Part model, mm, in its own coordinate system. Give positions to 0.01 mm unless a question says otherwise; leave off trailing zeros. Order: outer loops, then holes, each group sorted by start corner. A loop starts at its lowest first (then second) coordinate and runs counter-clockwise, first axis right, second up. Notation, with made-up numbers: M 45.25,28.5 L 52.25,28.5 A32 cw 52.25,64.5 Z; hole C 72,3 d10. An arc over 180 degrees is marked long. One line per question, with ' | ' between items.
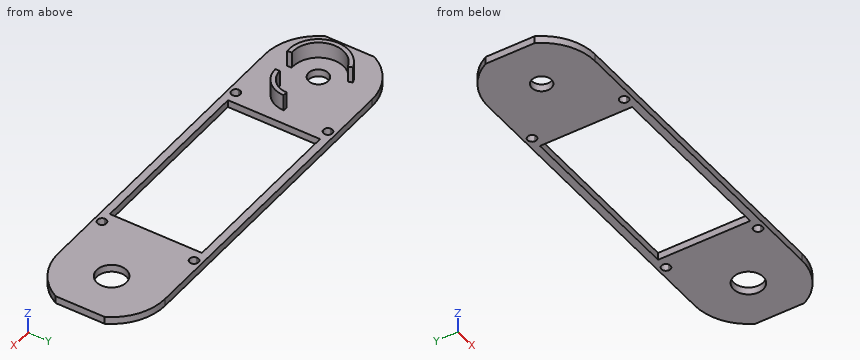
```python
from build123d import *

# Parameters (mm, degrees)
F0_R     = 30
F0_R_2   = 10
F0_R_3   = 14
F0_R_4   = 6.6
F1_DEPTH = 5
F3_DEPTH = 11


with BuildPart() as f1:
    # F0 (on Top) → F1 (new body)
    with BuildSketch(Plane.XY):
        with BuildLine():
            ThreePointArc((18.3030052177, -31), (31.2642622481, -17.8478543831), (36, 0))
            ThreePointArc((36, 0), (31.2978497092, 17.7888898917), (18.4197442455, 30.9307779069))
            ThreePointArc((18.4197442455, 30.9307779069), (9.5522770937, 34.7095664382), (0, 36))
            ThreePointArc((0, 36), (-18.7386337537, 30.7386337537), (-32, 16.4924225025))
            Line((-32, 16.4924225025), (-32, -16.4924225025))
            ThreePointArc((-32, -16.4924225025), (-18.7386337537, -30.7386337537), (0, -36))
            ThreePointArc((0, -36), (9.4868329805, -34.7275107084), (18.3030052177, -31))
        make_face()
        Circle(F0_R, mode=Mode.SUBTRACT)
        with BuildLine():
            ThreePointArc((242, 16.4924225025), (228.7386337537, 30.7386337537), (210, 36))
            ThreePointArc((210, 36), (200.4477229063, 34.7095664382), (191.5802557545, 30.9307779069))
            ThreePointArc((191.5802557545, 30.9307779069), (174.0000639573, -0.0678595955), (191.6969947823, -31))
            ThreePointArc((191.6969947823, -31), (200.5131670195, -34.7275107084), (210, -36))
            ThreePointArc((210, -36), (228.7386337537, -30.7386337537), (242, -16.4924225025))
            Line((242, -16.4924225025), (242, 16.4924225025))
        make_face()
        with Locations((210, 0)):
            Circle(F0_R, mode=Mode.SUBTRACT)
        Circle(F0_R)
        Circle(F0_R_2, mode=Mode.SUBTRACT)
        with Locations((210, 0)):
            Circle(F0_R)
        with Locations((210, 0)):
            Circle(F0_R_3, mode=Mode.SUBTRACT)
        with BuildLine():
            ThreePointArc((19.6214168703, 36), (23.4046464655, 33.6633706545), (26.9125802938, 30.9307779069))
            Line((26.9125802938, 30.9307779069), (34, 30.9307779069))
            ThreePointArc((34, 30.9307779069), (37, 33.9307779069), (40, 30.9307779069))
            Line((40, 30.9307779069), (45, 30.9307779069))
            Line((45, 30.9307779069), (165, 30.9307779069))
            Line((165, 30.9307779069), (170, 30.9307779069))
            ThreePointArc((170, 30.9307779069), (173, 33.9307779069), (176, 30.9307779069))
            Line((176, 30.9307779069), (183.0874197062, 30.9307779069))
            ThreePointArc((183.0874197062, 30.9307779069), (186.5953535345, 33.6633706545), (190.3785831296, 36))
            Line((190.3785831296, 36), (19.6214168703, 36))
        make_face()
        with BuildLine():
            Line((34, -31), (26.83281573, -31))
            ThreePointArc((26.83281573, -31), (23.361269906, -33.693487032), (19.6214168703, -36))
            Line((19.6214168703, -36), (190.3785831296, -36))
            ThreePointArc((190.3785831296, -36), (186.638730094, -33.693487032), (183.16718427, -31))
            Line((183.16718427, -31), (176, -31))
            ThreePointArc((176, -31), (173, -34), (170, -31))
            Line((170, -31), (165, -31))
            Line((165, -31), (45, -31))
            Line((45, -31), (40, -31))
            ThreePointArc((40, -31), (37, -34), (34, -31))
        make_face()
        with Locations((210, 0)):
            Circle(F0_R_3)
        with Locations((210, 0)):
            Circle(F0_R_2, mode=Mode.SUBTRACT)
        with BuildLine():
            Line((37, 27.9307779069), (37, 17.6635217327))
            ThreePointArc((37, 17.6635217327), (39.9874980463, 9.0553851381), (41, 0))
            ThreePointArc((41, 0), (39.9874980463, -9.0553851381), (37, -17.6635217327))
            Line((37, -17.6635217327), (37, -28))
            ThreePointArc((37, -28), (39.1213203436, -28.8786796564), (40, -31))
            Line((40, -31), (45, -31))
            Line((45, -31), (45, 30.9307779069))
            Line((45, 30.9307779069), (40, 30.9307779069))
            ThreePointArc((40, 30.9307779069), (39.1213203436, 28.8094575634), (37, 27.9307779069))
        make_face()
        with BuildLine():
            ThreePointArc((173, -17.6635217327), (169, 0), (173, 17.6635217327))
            Line((173, 17.6635217327), (173, 27.9307779069))
            ThreePointArc((173, 27.9307779069), (170.8786796564, 28.8094575634), (170, 30.9307779069))
            Line((170, 30.9307779069), (165, 30.9307779069))
            Line((165, 30.9307779069), (165, -31))
            Line((165, -31), (170, -31))
            ThreePointArc((170, -31), (170.8786796564, -28.8786796564), (173, -28))
            Line((173, -28), (173, -17.6635217327))
        make_face()
        Circle(F0_R_2)
        Circle(F0_R_4, mode=Mode.SUBTRACT)
        with BuildLine():
            ThreePointArc((18.4197442455, 30.9307779069), (31.2978497092, 17.7888898917), (36, 0))
            ThreePointArc((36, 0), (31.2642622481, -17.8478543831), (18.3030052177, -31))
            Line((18.3030052177, -31), (26.83281573, -31))
            ThreePointArc((26.83281573, -31), (32.6055594055, -24.8571417474), (37, -17.6635217327))
            Line((37, -17.6635217327), (37, 17.6635217327))
            ThreePointArc((37, 17.6635217327), (32.6375474194, 24.815126404), (26.9125802938, 30.9307779069))
            Line((26.9125802938, 30.9307779069), (18.4197442455, 30.9307779069))
        make_face()
        with BuildLine():
            Line((191.5802557545, 30.9307779069), (183.0874197062, 30.9307779069))
            ThreePointArc((183.0874197062, 30.9307779069), (177.3624525806, 24.815126404), (173, 17.6635217327))
            Line((173, 17.6635217327), (173, -17.6635217327))
            ThreePointArc((173, -17.6635217327), (177.3944405945, -24.8571417474), (183.16718427, -31))
            Line((183.16718427, -31), (191.6969947823, -31))
            ThreePointArc((191.6969947823, -31), (174.0000639573, -0.0678595955), (191.5802557545, 30.9307779069))
        make_face()
        with BuildLine():
            ThreePointArc((41, 0), (39.9874980463, 9.0553851381), (37, 17.6635217327))
            Line((37, 17.6635217327), (37, -17.6635217327))
            ThreePointArc((37, -17.6635217327), (39.9874980463, -9.0553851381), (41, 0))
        make_face()
        with BuildLine():
            Line((173, -17.6635217327), (173, 17.6635217327))
            ThreePointArc((173, 17.6635217327), (169, 0), (173, -17.6635217327))
        make_face()
        with BuildLine():
            ThreePointArc((0, 36), (9.5522770937, 34.7095664382), (18.4197442455, 30.9307779069))
            Line((18.4197442455, 30.9307779069), (26.9125802938, 30.9307779069))
            ThreePointArc((26.9125802938, 30.9307779069), (23.4046464655, 33.6633706545), (19.6214168703, 36))
            Line((19.6214168703, 36), (0, 36))
        make_face()
        with BuildLine():
            Line((210, 36), (190.3785831296, 36))
            ThreePointArc((190.3785831296, 36), (186.5953535345, 33.6633706545), (183.0874197062, 30.9307779069))
            Line((183.0874197062, 30.9307779069), (191.5802557545, 30.9307779069))
            ThreePointArc((191.5802557545, 30.9307779069), (200.4477229063, 34.7095664382), (210, 36))
        make_face()
        with BuildLine():
            Line((26.83281573, -31), (18.3030052177, -31))
            ThreePointArc((18.3030052177, -31), (9.4868329805, -34.7275107084), (0, -36))
            Line((0, -36), (19.6214168703, -36))
            ThreePointArc((19.6214168703, -36), (23.361269906, -33.693487032), (26.83281573, -31))
        make_face()
        with BuildLine():
            ThreePointArc((183.16718427, -31), (186.638730094, -33.693487032), (190.3785831296, -36))
            Line((190.3785831296, -36), (210, -36))
            ThreePointArc((210, -36), (200.5131670195, -34.7275107084), (191.6969947823, -31))
            Line((191.6969947823, -31), (183.16718427, -31))
        make_face()
        with BuildLine():
            ThreePointArc((37, -17.6635217327), (32.6055594055, -24.8571417474), (26.83281573, -31))
            Line((26.83281573, -31), (34, -31))
            ThreePointArc((34, -31), (34.8786796564, -28.8786796564), (37, -28))
            Line((37, -28), (37, -17.6635217327))
        make_face()
        with BuildLine():
            Line((176, -31), (183.16718427, -31))
            ThreePointArc((183.16718427, -31), (177.3944405945, -24.8571417474), (173, -17.6635217327))
            Line((173, -17.6635217327), (173, -28))
            ThreePointArc((173, -28), (175.1213203436, -28.8786796564), (176, -31))
        make_face()
        with BuildLine():
            Line((34, 30.9307779069), (26.9125802938, 30.9307779069))
            ThreePointArc((26.9125802938, 30.9307779069), (32.6375474194, 24.815126404), (37, 17.6635217327))
            Line((37, 17.6635217327), (37, 27.9307779069))
            ThreePointArc((37, 27.9307779069), (34.8786796564, 28.8094575634), (34, 30.9307779069))
        make_face()
        with BuildLine():
            ThreePointArc((173, 17.6635217327), (177.3624525806, 24.815126404), (183.0874197062, 30.9307779069))
            Line((183.0874197062, 30.9307779069), (176, 30.9307779069))
            ThreePointArc((176, 30.9307779069), (175.1213203436, 28.8094575634), (173, 27.9307779069))
            Line((173, 27.9307779069), (173, 17.6635217327))
        make_face()
    extrude(amount=F1_DEPTH)

    # F2 (on face) → F3 (join)
    with BuildSketch(Plane.XY.offset(5)):
        with BuildLine():
            ThreePointArc((32.2300370842, 0), (28.249548951, -9.6195118668), (18.6300370842, -13.6))
            Line((18.6300370842, -13.6), (18.6278837067, -16.5999992272))
            ThreePointArc((18.6278837067, -16.5999992272), (30.3708692945, -11.7408322103), (35.2300363114, 0.0021533775))
            Line((35.2300363114, 0.0021533775), (32.2300370842, 0))
        make_face()
        with BuildLine():
            ThreePointArc((1.4010723087, -16.9409777332), (-16.6169103502, -3.544385222), (-5.6333881929, 16.0382252023))
            Line((-5.6333881929, 16.0382252023), (-6.6291181037, 18.8681584073))
            ThreePointArc((-6.6291181037, 18.8681584073), (-19.550908877, -4.1702067977), (1.6467177805, -19.9309038698))
            Line((1.6467177805, -19.9309038698), (1.4010723087, -16.9409777332))
        make_face()
    extrude(amount=F3_DEPTH)


solid = f1.part
```
1. Slice it at C-C on y = -23. Give the cut face in (x, z).
Worked out:
outline: M -27.69,0 L 45,0 L 45,5 L -27.69,5 Z; M 165,0 L 237.69,0 L 237.69,5 L 165,5 Z
2. Slice it at A-A on x = 89. Give the cut face in (y, z).
Worked out:
outline: M -36,0 L -31,0 L -31,5 L -36,5 Z; M 30.93,0 L 36,0 L 36,5 L 30.93,5 Z
3. Slice it at B-B on y = 2.5. Give the cut face in (x, z).
Worked out:
outline: M -32,0 L -6.11,0 L -6.11,5 L -16.81,5 L -16.81,16 L -19.83,16 L -19.83,5 L -32,5 Z; M 6.11,0 L 45,0 L 45,5 L 6.11,5 Z; M 165,0 L 200.32,0 L 200.32,5 L 165,5 Z; M 219.68,0 L 242,0 L 242,5 L 219.68,5 Z
4. Slice it at D-D on x = 224. Give the cut face in (y, z).
Worked out:
outline: M -33.17,0 L 33.17,0 L 33.17,5 L -33.17,5 Z
5. Probe L1, parallel to Y at x = 210, z = 2.4; L2, parallel to Y at x = 0, z = 2.15; L3, parallel to Z at x = 229, y = 20.5. List the from-to ranges inside material, lowest first. Write a range as from..to.
Worked out:
L1: y = -36..-10, 10..36 | L2: y = -36..-6.6, 6.6..36 | L3: z = 0..5
6. Drop flat-ended pins along their axis: pin 1 (1.5 mm diameter, centred on x = 24, z = 12, fed in from -Y); pin 2 (6 mm diameter, centred on y = 5.5, z = 10, fed in from -X); pin 3 (1 mm diameter, centred on x = 201.5, y = -6.5, fed in from +Z). Give the stop position or say it passes through.
Worked out:
pin 1: stops at y = -15.95 | pin 2: stops at x = -19.83 | pin 3: stops at z = 5
